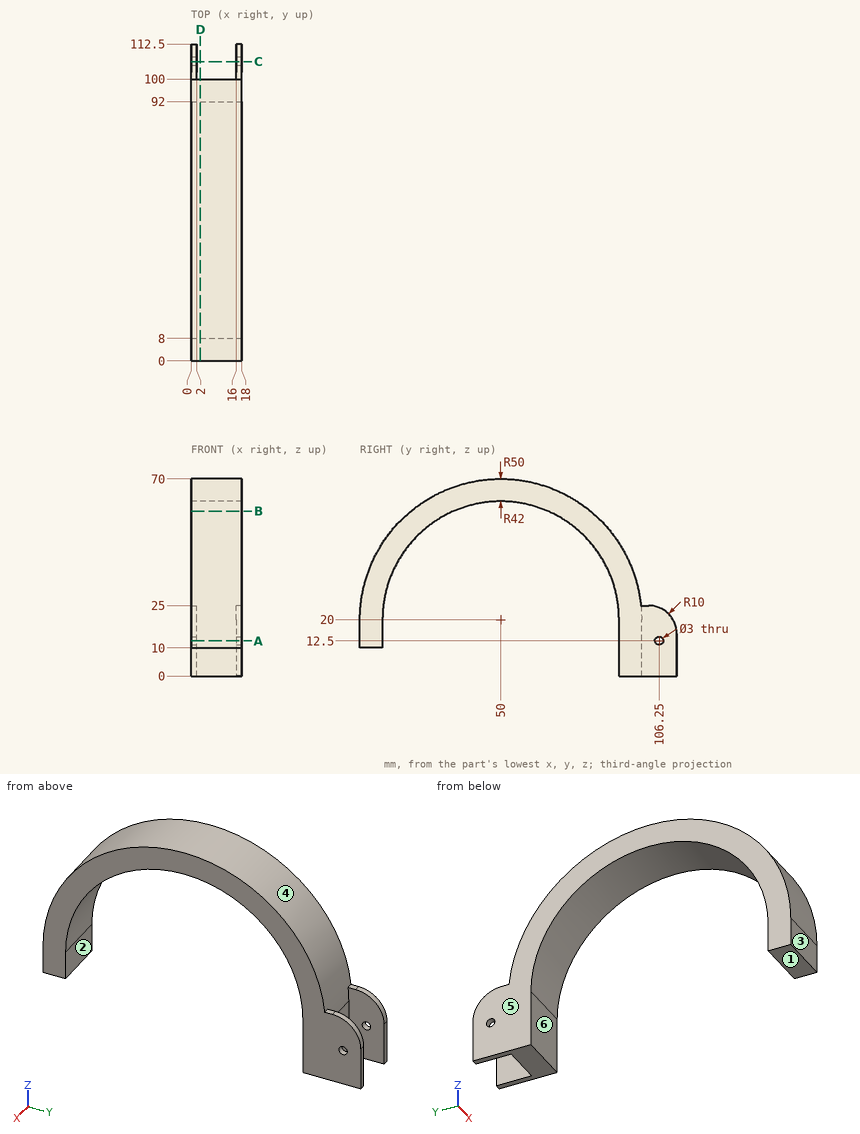
Study the drawing (mm; zero at the part's minimum x, y, z) and answer. A direction names the side the tool comes from. Round coordinates to 2 decimals unless told otherwise and drop trailing zeros. Order: outer loops, then holes, each group sorted by start corner. A loop starts at its lowest first (then second) coordinate and runs counter-clockwise, first axis right, second up. Notation, with made-up numbers: (-14, 57.5) -> (4, 57.5) arc R12 cw to (4, 62.5) -> close; hole circle Ø11 at (20.5, -39). An arc over 180 degrees is marked (long way). Write each question's results on one line, items separated by ' | '. Start each with the question number.
Q1. Each of these flat-tipped pins is pushed along its axis until it touches: pin 1 (2.5 mm diameter, centred on x = 12, y = 4.5, fed in from -Z); pin 2 (6 mm diameter, centred on x = 4.5, y = 37.5, fed in from +Z); pin 3 (6 mm diameter, centred on x = 11, y = 83, fed in from -Z). Where does it stop, or does it pass through?
Q2. Find section B-B (z = 58.5). Determine the outline of the cut face in (x, y), then the cut area to 3 significant figures.
Q3. Find section A-A (z = 12.5). Determine the outline of the cut face in (x, y).
Q4. The mould has two halves that part along Y. Classify the marked faces 1, 2, 3 and 4: pulls with the +Y half, pulls with the -Y half, needs draft (parallel to the pull), parting line crosses it, or undercut.
Q5. Find section C-C (y = 106.25). Determine the outline of the cut face in (x, z), then the cut area to 3 significant figures.
Q6. Straight lines are drawn through the part: probe 1 along Y at (x, z) = (0.95, 12.5); probe 2 along X at (y, z) = (102.5, 3); probe 3 along Y at (x, z) = (11.5, 16.5). For each, find the intervals that lie inside material, in ascending order. Write a range as from..to.
Q7. Find section D-D (x = 3.25). Determine the outline of the cut face in (y, z).
Q8. Which of the six approach directions +Z, -Z, +X, -X, +Y, -Y give full straight-line access (tool end or side, diameter ignored) to the marked faces 5 and 6?
Worked answers:
1) pin 1: stops at z = 10 | pin 2: stops at z = 69.09 | pin 3: stops at z = 41.63
2) outline: (0, 18.1) -> (18, 18.1) -> (18, 33.21) -> (0, 33.21) -> close; (0, 66.79) -> (18, 66.79) -> (18, 81.9) -> (0, 81.9) -> close | area: 544 mm2
3) outline: (0, 0) -> (18, 0) -> (18, 8) -> (0, 8) -> close; (0, 92) -> (18, 92) -> (18, 104.75) -> (16, 104.75) -> (16, 100) -> (2, 100) -> (2, 104.75) -> (0, 104.75) -> close; (0, 107.75) -> (2, 107.75) -> (2, 112.5) -> (0, 112.5) -> close; (16, 107.75) -> (18, 107.75) -> (18, 112.5) -> (16, 112.5) -> close
4) face 1: needs draft | face 2: undercut | face 3: pulls with the -Y half | face 4: parting line crosses it
5) outline: (0, 0) -> (2, 0) -> (2, 11) -> (0, 11) -> close; (0, 14) -> (2, 14) -> (2, 24.27) -> (0, 24.27) -> close; (16, 0) -> (18, 0) -> (18, 11) -> (16, 11) -> close; (16, 14) -> (18, 14) -> (18, 24.27) -> (16, 24.27) -> close | area: 85.1 mm2
6) probe 1: y = 0..8, 92..104.75, 107.75..112.5 | probe 2: x = 0..2, 16..18 | probe 3: y = 0..8, 92..100
7) outline: (0, 10) -> (8, 10) -> (8, 20) arc R42 cw to (92, 20) -> (92, 0) -> (100, 0) -> (100, 20) arc R50 ccw to (0, 20) -> close
8) face 5: +Z, -Z, -X, +Y, -Y | face 6: -Z, +X, -X
